```python
from build123d import *

# Parameters (mm, degrees)
F1_DEPTH = 19.05
F3_DEPTH = 19.05


# Not quite as in the source:
# - a feature names something its author has since deleted; it is built from what else it names


with BuildPart() as f1:
    # F0 (on Top) → F1 (new body)
    with BuildSketch(Plane.XY):
        Polygon((-39.6296493709, 39.737109375), (-44.4920025766, 39.737109375), (-45.0404509902, 38.3060877886), (-51.4150857925, 21.0715923085), (-52.2047057748, 19.1882997751), (-47.2585186362, 19.1882997751), (-46.5040132403, 21.2327073224), (-40.3436794877, 37.7105511725), align=None)
    extrude(amount=F1_DEPTH)



with BuildPart() as f1b:
    # F0 (on Top) → F1, piece 2 (new body)
    with BuildSketch(Plane.XY):
        Polygon((-52.8753772378, 39.737109375), (-58.071937412, 39.737109375), (-65.8153370023, 19.1017910838), (-61.0744804144, 19.1017910838), (-57.5978495181, 27.8723798692), (-58.2299642265, 19.1017910838), (-52.9360063374, 19.1017910838), (-52.2047057748, 21.0715923085), (-45.9454512168, 38.3060877886), (-45.4141758382, 39.737109375), (-49.9411970377, 39.737109375), (-53.4955092069, 30.7705519863), align=None)
    extrude(amount=F1_DEPTH)


with BuildPart() as f1c:
    # F0 (on Top) → F1, piece 3 (new body)
    with BuildSketch(Plane.XY):
        with BuildLine():
            Line((-34.012787044, 39.737109375), (-38.875143975, 39.737109375))
            Line((-38.875143975, 39.737109375), (-39.4490547478, 37.7105511725))
            Line((-39.4490547478, 37.7105511725), (-45.7450146313, 21.2327073224))
            Line((-45.7450146313, 21.2327073224), (-46.5040132403, 19.1882997751))
            Line((-46.5040132403, 19.1882997751), (-41.5926604458, 18.9808556717))
            Line((-41.5926604458, 18.9808556717), (-38.3721441031, 27.6555065066))
            Line((-38.3721441031, 27.6555065066), (-38.1206423044, 19.1044658422))
            Line((-38.1206423044, 19.1044658422), (-31.3301086426, 19.1044658422))
            Line((-31.3301086426, 19.1044658422), (-57.9053983092, 11.8109323084))
            ThreePointArc((-57.9053983092, 11.8109323084), (-61.6554191389, 11.565355508), (-65.1989355683, 12.816936709))
            ThreePointArc((-65.1989355683, 12.816936709), (-67.1816299808, 14.8061054603), (-68.3846175671, 17.3439569771))
            ThreePointArc((-68.3846175671, 17.3439569771), (-68.0426528163, 21.7039427005), (-66.5402710438, 25.8111637086))
            ThreePointArc((-66.5402710438, 25.8111637086), (-68.289988101, 23.8168641952), (-69.8936209083, 21.7033121735))
            ThreePointArc((-69.8936209083, 21.7033121735), (-71.9777744598, 18.6120372362), (-73.74997437, 15.331948176))
            ThreePointArc((-73.74997437, 15.331948176), (-75.226699634, 12.199885885), (-76.2, 8.8767521083))
            ThreePointArc((-76.2, 8.8767521083), (-76.0035829361, 5.2955374253), (-73.74997437, 2.505389275))
            ThreePointArc((-73.74997437, 2.505389275), (-69.4068023904, 0.267420013), (-64.5282641053, 0))
            Line((-64.5282641053, 0), (-58.5760697722, 1.9185534911))
            Line((-58.5760697722, 1.9185534911), (0, 27.1525029093))
            Line((0, 27.1525029093), (-22.3599020392, 21.367976442))
            Line((-22.3599020392, 21.367976442), (-21.9407342374, 23.0446513742))
            Line((-21.9407342374, 23.0446513742), (-27.3060910404, 23.0446513742))
            Line((-27.3060910404, 23.0446513742), (-25.5455821753, 27.9908403754))
            Line((-25.5455821753, 27.9908403754), (-20.9347270429, 27.9908403754))
            Line((-20.9347270429, 27.9908403754), (-19.4257199764, 31.9310240448))
            Line((-19.4257199764, 31.9310240448), (-24.2042429745, 31.9310240448))
            Line((-24.2042429745, 31.9310240448), (-22.5275680423, 36.2903773785))
            Line((-22.5275680423, 36.2903773785), (-17.5813790411, 36.2903773785))
            Line((-17.5813790411, 36.2903773785), (-16.2400398403, 39.737109375))
            Line((-16.2400398403, 39.737109375), (-30.827106908, 39.737109375))
            Line((-30.827106908, 39.737109375), (-36.0247977078, 33.607698977))
            Line((-36.0247977078, 33.607698977), (-34.012787044, 39.737109375))
        make_face()
        Polygon((-26.2162536383, 38.9730595052), (-33.3421193063, 20.5296389759), (-33.7612889707, 31.1765223742), align=None, mode=Mode.SUBTRACT)
    extrude(amount=F1_DEPTH)


with BuildPart() as f1_1:
    add(f1.part)

    add(f1b.part)  # F3 merges F1b

    add(f1c.part)  # F3 merges F1c
    # F2 (on Top) → F3 (join, through all)
    with BuildSketch(Plane.XY):
        Polygon((-39.4490547478, 37.7105511725), (-38.875143975, 39.737109375), (-39.6296493709, 39.737109375), (-40.3436794877, 37.7105511725), align=None)
        Polygon((-46.5040132403, 19.1882997751), (-45.7450146313, 21.2327073224), (-46.5040132403, 21.2327073224), (-47.2585186362, 19.1882997751), align=None)
        Polygon((-52.2047057748, 19.1882997751), (-51.4150857925, 21.0715923085), (-52.2047057748, 21.0715923085), (-52.9360063374, 19.1017910838), align=None)
        Polygon((-45.0404509902, 38.3060877886), (-44.4920025766, 39.737109375), (-45.4141758382, 39.737109375), (-45.9454512168, 38.3060877886), align=None)
    extrude(amount=F3_DEPTH)


solid = f1_1.part
```
Can you work these out from the model? Positions are in its coordinate system, mm. A direction names the side the tool comes from. Coordinates: 2 decimals unless noted, no trailing zeros. Loops run counter-clockwise (first coordinate to the right, second up) from the corner with the lowest first, then second, coordinate; pieces in that order, holes last. Notation, with made-up numbers: (-12.5, 10) - (-6.5, 10) arc R17 cw to (-6.5, 42) - close; hole circle Ø10 at (-18, 75). An arc over 180 degrees is marked (long way). Answer as CSV lines item,"result". Start each with the question number.
1) Which directions (+Z, -Z, +X, -X, +Y, -Y) give clear straight access to the entire face, cutting with the end or side of a thin tool? Please do faces 4 (the flat face through (-49, 19.188, 9)), 5 (the cylindrical face through (-68.266, 23.846, 9.392)), 6 (the flat face through (-22, 31.931, 9)).
2) Suppose I cut it at D-D (y = 4). Please give me the cut outline in (x, z).
3) I need wall thicknesses on line 1 (X direction, y = 33, z = 10); line 2 (X direction, y = 35, z = 11.25); line 3 (X direction, y = 31.5, z = 18). Which ranges of each line are inside material? Lowest first, please. Write a range as from..to.
4) Suppose I cut it at B-B (z = 14.75). Count the separate pieces of the cut face and the enclosed holes in it, plus the area to 3 significant figures.
5) Thinking about a two-plate mould opening in X: for faces 1 (the flat face through (-23, 27.991, 9)), 2 (the flat face through (-35, 19.104, 9)), 3 (the cylindrical face through (-71.95, 18.66, 9.39)), which applies, pulls with the +X half, pulls with the -X half, needs draft (parallel to the pull), parting line crosses it, or undercut?
6) For pin 1 (4 mm diameter, centred on x = -56.5, z = 10.5, fed in from -Y); pin 2 (1 mm diameter, centred on y = 29.5, z = 11, fed in from -X); pin 3 (5 mm diameter, centred on x = -63.5, z = 8, fed in from -Y), each with a flat end and sliding along its axis, tell me the tip position at first contact or that it passes through.
7) Suppose I cut it at A-A (x = -28.5). Please give me the cut outline in (y, z) (3 decimals), plus the area to 3 significant figures.
8) Suppose I cut it at C-C (x = -62.5). Please give me the cut outline in (y, z), plus the area to 3 significant figures.
Check result:
1,face 4,"+Z, -Z"
1,face 5,"+Z, -Z, -X, +Y"
1,face 6,"+Z, -Z, +X"
2,outline,"(-75.31, 0) - (-53.74, 0) - (-53.74, 19.05) - (-75.31, 19.05) - close"
3,line 1,"x = -60.6..-53.34, -52.61..-47.87, -47..-42.1, -41.25..-32, -28.52..-23.79"
3,line 2,"x = -59.85..-53.2, -51.82..-47.15, -46.26..-41.36, -40.48..-35.57, -34.84..-30.06, -27.75..-23.02"
3,line 3,"x = -61.16..-53.45, -53.21..-48.42, -47.56..-42.67, -41.82..-33.45, -29.1..-19.59"
4,separate pieces,"1"
4,enclosed holes,"3"
4,area,"1,230 mm²"
5,face 1,"needs draft"
5,face 2,"undercut"
5,face 3,"pulls with the -X half"
6,pin 1,"stops at y = 1.95"
6,pin 2,"stops at x = -62.1"
6,pin 3,"stops at y = -0.14"
7,outline,"(14.875, 0) - (33.062, 0) - (33.062, 19.05) - (14.875, 19.05) - close; (36.613, 0) - (39.737, 0) - (39.737, 19.05) - (36.613, 19.05) - close"
7,area,"406 mm²"
8,outline,"(0.65, 0) - (11.72, 0) - (11.72, 19.05) - (0.65, 19.05) - close; (19.1, 0) - (27.94, 0) - (27.94, 19.05) - (19.1, 19.05) - close"
8,area,"379 mm²"
